The listing builds one solid part. Answer for the finished solid, in the listing's coordinates (mm). Face numbers are marked on the shaded views. A direction names the side the tool comes from. Round coordinates to 2 decimals unless told otherwise and drop trailing zeros. Write each loop counter-clockwise with the first axis right and the second up, starting at its lowest first coordinate (ties: lowest second). Pieces come first, ordered by that corner, then holes. Notation, with made-up numbers: M 48,-7.75 L 73,-7.75 A21 ccw 73,-3.75 Z; hole C 15,21.25 d5. An arc over 180 degrees is marked long. Write each question's results on one line, items separated by ' | '.
from build123d import *

# Parameters (mm, degrees)
SKETCH_1_R          = 7.5
SKETCH_1_R_2        = 3
EXTRUDE_1_DEPTH     = 3
SKETCH_2_R          = 7.5
SKETCH_2_R_2        = 1.8
EXTRUDE_2_DEPTH     = 3.5
SKETCH_3_R          = 5.75
SKETCH_3_R_2        = 4
CUT_EXTRUDE_1_DEPTH = 2
SKETCH_4_R          = 4
SKETCH_4_R_2        = 1.7
EXTRUDE_3_DEPTH     = 4
SKETCH_5_R          = 3
CUT_EXTRUDE_2_DEPTH = 3.5
CHAMFER_1_SIZE      = 0.6


with BuildPart() as part:
    # Эскиз1 → Бобышка-Вытянуть1 (new body)
    with BuildSketch(Plane(origin=(0, 0, 0), x_dir=(1, 0, 0), z_dir=(0, 1, 0))):
        with Locations((-2.5, 0)):
            Circle(SKETCH_1_R)
        Circle(SKETCH_1_R_2, mode=Mode.SUBTRACT)
    extrude(amount=EXTRUDE_1_DEPTH)

    # Эскиз2 → Бобышка-Вытянуть2 (add)
    with BuildSketch(Plane(origin=(0, 3, 0), x_dir=(1, 0, 0), z_dir=(0, 1, 0))):
        with Locations((-2.5, 0)):
            Circle(SKETCH_2_R)
        Circle(SKETCH_2_R_2, mode=Mode.SUBTRACT)
    extrude(amount=EXTRUDE_2_DEPTH)

    # Эскиз3 → Вырез-Вытянуть1 (cut)
    with BuildSketch(Plane(origin=(0, 6.5, 0), x_dir=(1, 0, 0), z_dir=(0, 1, 0))):
        Circle(SKETCH_3_R)
        Circle(SKETCH_3_R_2, mode=Mode.SUBTRACT)
    extrude(amount=-CUT_EXTRUDE_1_DEPTH, mode=Mode.SUBTRACT)

    # Эскиз4 → Бобышка-Вытянуть3 (add)
    with BuildSketch(Plane(origin=(0, 6.5, 0), x_dir=(1, 0, 0), z_dir=(0, 1, 0))):
        Circle(SKETCH_4_R)
        Circle(SKETCH_4_R_2, mode=Mode.SUBTRACT)
    extrude(amount=EXTRUDE_3_DEPTH)

    # Эскиз5 → Вырез-Вытянуть2 (cut)
    with BuildSketch(Plane.XZ):
        Circle(SKETCH_5_R)
    extrude(amount=-CUT_EXTRUDE_2_DEPTH, mode=Mode.SUBTRACT)

    # Фаска1
    chamfer_1_edges = [part.edges().sort_by_distance(p)[0] for p in [
        (-3, 0, 0),
    ]]
    chamfer(chamfer_1_edges, length=CHAMFER_1_SIZE)


solid = part.part
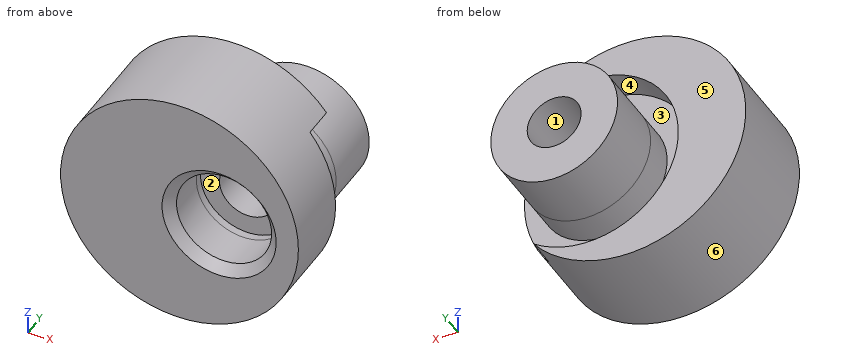
1) Section C-C (y = 7) is taken. Determine the outline of the cut face in (x, z), then the cut area to 3 significant figures.
Return value:
outline: C 0,0 d8; hole C 0,0 d3.4 | area: 41.2 mm²
2) The mould has two halves that part along X. Classify the marked faces 4, 5 and 6: +X half, -X half, draft (parallel to the pull), parting line (faces both ways), or undercut.
Return value:
face 4: undercut | face 5: draft | face 6: parting line
3) Section B-B (x = 0) is taken. Determine the outline of the cut face in (y, z), then the cut area to 3 significant figures.
Return value:
outline: M 0,-7.07 L 6.5,-7.07 L 6.5,-5.75 L 4.5,-5.75 L 4.5,-4 L 10.5,-4 L 10.5,-1.7 L 6.5,-1.7 L 6.5,-1.8 L 3.5,-1.8 L 3.5,-3 L 0.6,-3 L 0,-3.6 Z; M 0,3.6 L 0.6,3 L 3.5,3 L 3.5,1.8 L 6.5,1.8 L 6.5,1.7 L 10.5,1.7 L 10.5,4 L 4.5,4 L 4.5,5.75 L 6.5,5.75 L 6.5,7.07 L 0,7.07 Z | area: 71.2 mm²
4) Each of these flat-tipped pins is pushed along its axis until it touches: pin 1 (5 mm diameter, centred on x = 0, z = 0, fed in from -Y); pin 2 (3 mm diameter, centred on x = 0, y = 2.5, fed in from -Z); pin 3 (6 mm diameter, centred on y = 3.5, z = -4, fed in from +X). Where does it stop, or does it pass through?
Return value:
pin 1: y = 3.5 | pin 2: z = -7.43 | pin 3: x = 4.93
5) Find the intervals of material crossed by line 1 (X direction, y = 5.1, z = 0); line 2 (X direction, y = 9.4, z = 0); line 3 (X direction, y = 3.2, z = 0), in increasing order.
Return value:
line 1: -10 to -5.75, -4 to -1.8, 1.8 to 4 | line 2: -4 to -1.7, 1.7 to 4 | line 3: -10 to -3, 3 to 5
6) A tool of negligible diameter and unlimited length cuts with its end or side. For the marked faces 1, 2 and 3, from which of +Z, -Z, +X, -X, +Y, -Y can it reach the whole face along a straight path? Write none if from no direction.
Return value:
face 1: +Y, -Y | face 2: -Y | face 3: +Y
7) Section D-D (x = -4.75) is taken. Determine the outline of the cut face in (y, z), then the cut area to 3 significant figures.
Return value:
outline: M 0,-7.15 L 6.5,-7.15 L 6.5,-3.24 L 4.5,-3.24 L 4.5,3.24 L 6.5,3.24 L 6.5,7.15 L 0,7.15 Z | area: 80.0 mm²
8) Section A-A (z = 0) is taken. Determine the outline of the cut face in (x, y), then the cut area to 3 significant figures.
Return value:
outline: M -10,0 L -3.6,0 L -3,0.6 L -3,3.5 L -1.8,3.5 L -1.8,6.5 L -1.7,6.5 L -1.7,10.5 L -4,10.5 L -4,4.5 L -5.75,4.5 L -5.75,6.5 L -10,6.5 Z; M 1.7,6.5 L 1.8,6.5 L 1.8,3.5 L 3,3.5 L 3,0.6 L 3.6,0 L 5,0 L 5,4.5 L 4,4.5 L 4,10.5 L 1.7,10.5 Z | area: 78.2 mm²
